```python
from build123d import *

# Parameters (mm, degrees)
ESQUISSE1_R                    = 4.5
ESQUISSE1_R_2                  = 4
BOSS_EXTRU_1_DEPTH             = 28
BOSS_EXTRU_2_REACH             = 6.5
ESQUISSE2_R                    = 1
ESQUISSE2_R_2                  = 0.5
BOSS_EXTRU_2_DIRECTION_2_REACH = 6.5
ENL_V_MAT_EXTRU_1_DEPTH        = 5.5
ENL_V_MAT_EXTRU_1_DEPTH_BACK   = 5.5
ESQUISSE4_R                    = 3.5
BOSS_EXTRU_3_DEPTH             = 1
ESQUISSE6_OUTSIDE_W            = 31.274
ESQUISSE6_OUTSIDE_H            = 45.274
ESQUISSE6_OUTSIDE_W_2          = 16
ESQUISSE6_OUTSIDE_H_2          = 27
ENL_V_MAT_EXTRU_2_DEPTH        = 58.0000001
BOSS_EXTRU_6_START             = -1.5
ESQUISSE7_R                    = 1.45
BOSS_EXTRU_6_DEPTH             = 1
BOSS_EXTRU_7_REACH             = 23.5
BOSS_EXTRU_7_START             = 1
ESQUISSE8_R                    = 1.45
ENL_V_MAT_EXTRU_3_DEPTH        = 6
ENL_V_MAT_EXTRU_3_DEPTH_BACK   = 23


with BuildPart() as part:
    # Esquisse1 → Boss.-Extru.1 (new body, symmetric)
    with BuildSketch(Plane.XY):
        Circle(ESQUISSE1_R)
        Circle(ESQUISSE1_R_2, mode=Mode.SUBTRACT)
    extrude(amount=BOSS_EXTRU_1_DEPTH, both=True)

    # Esquisse2 → Boss.-Extru.2 (add, up to next)
    with BuildSketch(Plane(origin=(0, 0, 0), x_dir=(1, 0, 0), z_dir=(0, 1, 0)), mode=Mode.PRIVATE) as boss_extru_2_sk1:
        with Locations((0, -26.5)):
            Circle(ESQUISSE2_R)
    boss_extru_2_tool1 = extrude(boss_extru_2_sk1.sketch, amount=BOSS_EXTRU_2_REACH, mode=Mode.PRIVATE) - part.part
    add(boss_extru_2_tool1.solids().sort_by_distance((0, 0, 26.5))[0])
    # Esquisse2 → Boss.-Extru.2 (add, up to next)
    with BuildSketch(Plane(origin=(0, 0, 0), x_dir=(1, 0, 0), z_dir=(0, 1, 0)), mode=Mode.PRIVATE) as boss_extru_2_sk2:
        with Locations((3, 26.5)):
            Circle(ESQUISSE2_R_2)
    boss_extru_2_tool2 = extrude(boss_extru_2_sk2.sketch, amount=BOSS_EXTRU_2_REACH, mode=Mode.PRIVATE) - part.part
    add(boss_extru_2_tool2.solids().sort_by_distance((3, 0, -26.5))[0])

    # Esquisse2 → Boss.-Extru.2 direction 2 (add, up to next)
    with BuildSketch(Plane(origin=(0, 0, 0), x_dir=(1, 0, 0), z_dir=(0, 1, 0)), mode=Mode.PRIVATE) as boss_extru_2_direction_2_sk1:
        with Locations((0, -26.5)):
            Circle(ESQUISSE2_R)
    boss_extru_2_direction_2_tool1 = extrude(boss_extru_2_direction_2_sk1.sketch, amount=-BOSS_EXTRU_2_DIRECTION_2_REACH, mode=Mode.PRIVATE) - part.part
    add(boss_extru_2_direction_2_tool1.solids().sort_by_distance((0, 0, 26.5))[0])
    # Esquisse2 → Boss.-Extru.2 direction 2 (add, up to next)
    with BuildSketch(Plane(origin=(0, 0, 0), x_dir=(1, 0, 0), z_dir=(0, 1, 0)), mode=Mode.PRIVATE) as boss_extru_2_direction_2_sk2:
        with Locations((3, 26.5)):
            Circle(ESQUISSE2_R_2)
    boss_extru_2_direction_2_tool2 = extrude(boss_extru_2_direction_2_sk2.sketch, amount=-BOSS_EXTRU_2_DIRECTION_2_REACH, mode=Mode.PRIVATE) - part.part
    add(boss_extru_2_direction_2_tool2.solids().sort_by_distance((3, 0, -26.5))[0])

    # Esquisse3 → Enlèv. mat.-Extru.1 (cut, two sides)
    with BuildSketch(Plane(origin=(0, 0, 0), x_dir=(1, 0, 0), z_dir=(0, 1, 0))) as enl_v_mat_extru_1_sk:
        with BuildLine():
            Line((1, 28), (1, -24))
            ThreePointArc((1, -24), (0, -25), (-1, -24))
            Line((-1, -24), (-1, 28))
            ThreePointArc((-1, 28), (0, 29), (1, 28))
        make_face()
    extrude(amount=ENL_V_MAT_EXTRU_1_DEPTH, mode=Mode.SUBTRACT)
    extrude(enl_v_mat_extru_1_sk.sketch, amount=-ENL_V_MAT_EXTRU_1_DEPTH_BACK, mode=Mode.SUBTRACT)

    # Esquisse4 → Boss.-Extru.3 (add)
    with BuildSketch(Plane.XY.offset(28)):
        with BuildLine():
            Line((8, 0), (8, -14))
            ThreePointArc((8, -14), (0, -22), (-8, -14))
            Line((-8, -14), (-8, 0))
            ThreePointArc((-8, 0), (0, 8), (8, 0))
        make_face()
        Circle(ESQUISSE4_R, mode=Mode.SUBTRACT)
    extrude(amount=BOSS_EXTRU_3_DEPTH)

    # Esquisse6 outside → Enlèv. mat.-Extru.2 (cut, through all)
    with BuildSketch(Plane.XY.offset(29)):
        with Locations((0, -7)):
            Rectangle(ESQUISSE6_OUTSIDE_W, ESQUISSE6_OUTSIDE_H)
        with Locations((0, -8.5)):
            Rectangle(ESQUISSE6_OUTSIDE_W_2, ESQUISSE6_OUTSIDE_H_2, mode=Mode.SUBTRACT)
    extrude(amount=-ENL_V_MAT_EXTRU_2_DEPTH, mode=Mode.SUBTRACT)

    # Esquisse7 → Boss.-Extru.6 (add)
    with BuildSketch(Plane(origin=(0, 0, 0), x_dir=(1, 0, 0), z_dir=(0, 1, 0)).offset(BOSS_EXTRU_6_START)):
        with Locations((0, -26.5)):
            Circle(ESQUISSE7_R)
    extrude(amount=BOSS_EXTRU_6_DEPTH)

    # Esquisse8 → Boss.-Extru.7 (add, up to next)
    with BuildSketch(Plane.XZ.offset(1.5).offset(BOSS_EXTRU_7_START), mode=Mode.PRIVATE) as boss_extru_7_sk1:
        with Locations((0, 26.5)):
            Circle(ESQUISSE8_R)
    boss_extru_7_tool1 = extrude(boss_extru_7_sk1.sketch, amount=BOSS_EXTRU_7_REACH, mode=Mode.PRIVATE) - part.part
    add(boss_extru_7_tool1.solids().sort_by_distance((0, -2.5, 26.5))[0])

    # Esquisse9 → Enlèv. mat.-Extru.3 (cut, two sides)
    with BuildSketch(Plane(origin=(0, 0, 0), x_dir=(1, 0, 0), z_dir=(0, 1, 0))) as enl_v_mat_extru_3_sk:
        with BuildLine():
            Line((0, 25.4), (-3, 25.4))
            ThreePointArc((-3, 25.4), (-3.707106781, 25.692893219), (-4, 26.4))
            Line((-4, 26.4), (-4, 28))
            Line((-4, 28), (1.6, 28))
            Line((1.6, 28), (1.6, 27))
            ThreePointArc((1.6, 27), (1.13137085, 25.86862915), (0, 25.4))
        make_face()
    extrude(amount=ENL_V_MAT_EXTRU_3_DEPTH, mode=Mode.SUBTRACT)
    extrude(enl_v_mat_extru_3_sk.sketch, amount=-ENL_V_MAT_EXTRU_3_DEPTH_BACK, mode=Mode.SUBTRACT)


solid = part.part
```
Geometry: final body of the model. Coordinates: model frame, mm. A direction names the side the tool comes from. Round coordinates to 2 decimals unless told otherwise and drop trailing zeros. Order: outer loops, then holes, each group sorted by start corner. A loop starts at its lowest first (then second) coordinate and runs counter-clockwise, first axis right, second up. Notation, with made-up numbers: (-0.5, -2.5) -> (56.5, -2.5) arc R9 ccw to (56.5, 10.5) -> close; hole circle Ø5 at (35, -19). An arc over 180 degrees is marked (long way). Use CSV: the item, a comma, the result in double quotes. Start each with the question number.
1) Section C-C (y = 0.75). Return the cut outline in (x, z).
2) Section D-D (z = 26.5). Return the cut outline in (x, y), and give its area (3 significant figures).
3) Draft query along Y for faces 5 (the face through (-0.1, 5, 28.5)), 6 (the face through (-4, 0, -27)), 7 (the face through (3.695, -1.532, -0.392)). Return one class per face: +Y half, -Y half, draft (parallel to the pull), parting line (faces both ways), or undercut.
4) Material intervals for line 1 along X through (y, z) = (0, 9.5); line 2 along Y through (x, z) = (0, 28.35); line 3 along Z through (x, y) = (-5.75, -3.5), sorted ascending. Write a range as from..to.
5) Set-up query: faces 1 (the face through (4.292, 1.352, 0.392)), 2 (the face through (-8, -7.1, 28.5)), 3 (the face through (0.46, -2.01, 27.39)), 4 (the face through (-2.1, -3.6, -25.4)). Return all of +Z, -Z, +X, -X, +Y, -Y with unobstructed straight access to the full face (end or side cutting, diameter ignored); none if empty.
6) First-contact query: pin 1 Ø6 at (x, z) = (-2.5, 11.5) entering from +Y; pin 2 Ø2 at (x, y) = (6.5, -1.5) entering from -Z; pin 3 Ø3 at (x, z) = (0.5, 26) entering from +Y. Flat tips, straight axial feed; report the tip coordinate or a pass-through.
7) Section A-A (z = -21). Return the cut outline in (x, y).
Returned:
1,outline,"(-7.96, 28) -> (-4.44, 28) -> (-4.44, -28) -> (-4, -28) -> (-4, -26.4) arc R1 cw to (-3.93, -26.03) -> (-3.93, 28) -> (-3.42, 28) -> (-3.42, 29) -> (-7.96, 29) -> close; circle Ø2 at (0, 26.5); circle Ø1 at (3, -26.5); (3.42, 28) -> (3.93, 28) -> (3.93, -28) -> (4.44, -28) -> (4.44, 28) -> (7.96, 28) -> (7.96, 29) -> (3.42, 29) -> close"
2,outline,"circle Ø9 at (0, 0); hole (-1.45, -3.73) -> (-1.45, -2.5) -> (-1, -2.5) -> (-1, -1.5) -> (-1.45, -1.5) -> (-1.45, -0.5) -> (-1, -0.5) -> (-1, 3.87) arc R4 ccw to start; hole (1, -2.5) -> (1.45, -2.5) -> (1.45, -3.73) arc R4 ccw to (1, 3.87) -> (1, -0.5) -> (1.45, -0.5) -> (1.45, -1.5) -> (1, -1.5) -> close"
2,area,"31.3 mm²"
3,face 5,"+Y half"
3,face 6,"draft"
3,face 7,"undercut"
4,line 1,"x = -4.5..-4, 4..4.5"
4,line 2,"y = -22..-3.5, 3.5..5"
4,line 3,"z = 28..29"
5,face 1,"-Z"
5,face 2,"+Z, -Z, -X, +Y, -Y"
5,face 3,"none"
5,face 4,"-Z, +Y, -Y"
6,pin 1,"stops at y = 4.39"
6,pin 2,"stops at z = 28"
6,pin 3,"stops at y = 4.5"
7,outline,"(-1, -4.39) -> (-1, -3.87) arc R4 cw to (-1, 3.87) -> (-1, 4.39) arc R4.5 ccw to start; (1, -4.39) arc R4.5 ccw to (1, 4.39) -> (1, 3.87) arc R4 cw to (1, -3.87) -> close"
